from build123d import *

# Parameters (mm, degrees)
F0_W     = 50.8
F0_H     = 25.4
F1_DEPTH = 38.1
F3_DEPTH = 12.7


# Not quite as in the source:
# - a length typed as a fraction of an inch, garbled in the dataset ("3 / 203.2 mm" for 3/8 in), is restored


with BuildPart() as f1:
    # F0 (on Front) → F1 (new body)
    with BuildSketch(Plane.XZ):
        with Locations((-40.7616753732, 12.7)):
            Rectangle(F0_W, F0_H)
    extrude(amount=F1_DEPTH)

    # F2 (on face) → F3 (cut)
    with BuildSketch(Plane.XY.offset(25.4)):
        Polygon((-15.3616753732, 0), (-40.7616753732, 0), (-59.8116753732, -38.1), (-28.0616753732, -38.1), (-15.3616753732, -19.05), align=None)
    extrude(amount=-F3_DEPTH, mode=Mode.SUBTRACT)


solid = f1.part
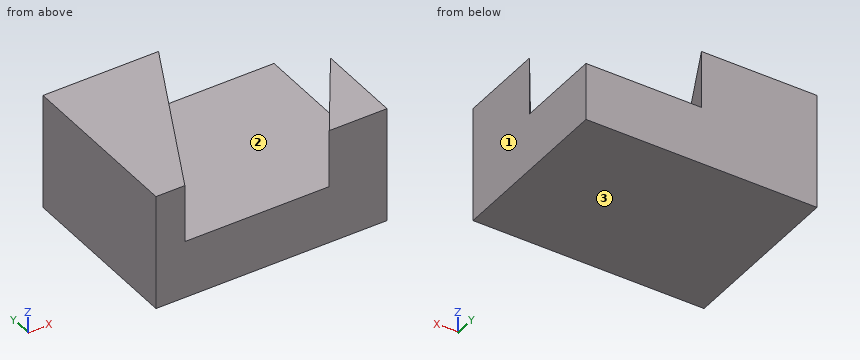
Source: CAD feature listing. Evaluate the final solid. Frame: model axes, mm. Face numbers are marked on the shaded views. Coordinates: 2 decimals unless noted, no trailing zeros. Order: outer loops, then holes, each group sorted by start corner. A loop starts at its lowest first (then second) coordinate and runs counter-clockwise, first axis right, second up. Notation, with made-up numbers: M -9.75,7 L 40.25,7 A21 cw 40.25,15 Z; hole C -14,42 d9. An arc over 180 degrees is marked long. Write each question's results on one line, items separated by ' | '. Start each with the question number.
1. Draft query along X for the marked faces 1, 2 and 3. Return one class per face: +X half, -X half, draft (parallel to the pull), parting line (faces both ways), or undercut.
2. Section C-C, the plane y = -9. Return the cut outline in (x, z).
3. Section B-B, the plane x = -38. Return the cut outline in (y, z).
4. Section D-D, the plane x = -50. Return the cut outline in (y, z), then the cut area to 3 significant figures.
5. Pin query (flat end, axial travel): pin 1 (4 mm diameter, centred on x = -31.5, y = -6.5, fed in from +Z); pin 2 (3 mm diameter, centred on y = -17.5, z = 14.5, fed in from +X). Return the tip coordinate at first contact, or that it passes through.
6. Section A-A, the plane z = 17. Return the cut outline in (x, y).
7. Material intervals for L1, parallel to Z at x = -35, y = -34.5; L2, parallel to X at y = -22.5, z = 19.25; L3, parallel to X at y = -27.5, z = 18.5 (3 decimals), sorted ascending.
Solution:
1) face 1: +X half | face 2: undercut | face 3: draft
2) outline: M -66.16,0 L -15.36,0 L -15.36,12.7 L -45.26,12.7 L -45.26,25.4 L -66.16,25.4 Z
3) outline: M -38.1,0 L 0,0 L 0,12.7 L -38.1,12.7 Z
4) outline: M -38.1,0 L 0,0 L 0,25.4 L -18.48,25.4 L -18.48,12.7 L -38.1,12.7 Z | area: 719 mm²
5) pin 1: z = 12.7 | pin 2: x = -48.76
6) outline: M -66.16,-38.1 L -59.81,-38.1 L -40.76,0 L -66.16,0 Z; M -28.06,-38.1 L -15.36,-38.1 L -15.36,-19.05 Z
7) L1: 0 to 12.7 | L2: -66.16 to -52.01, -17.66 to -15.36 | L3: -66.162 to -54.512, -20.995 to -15.362
